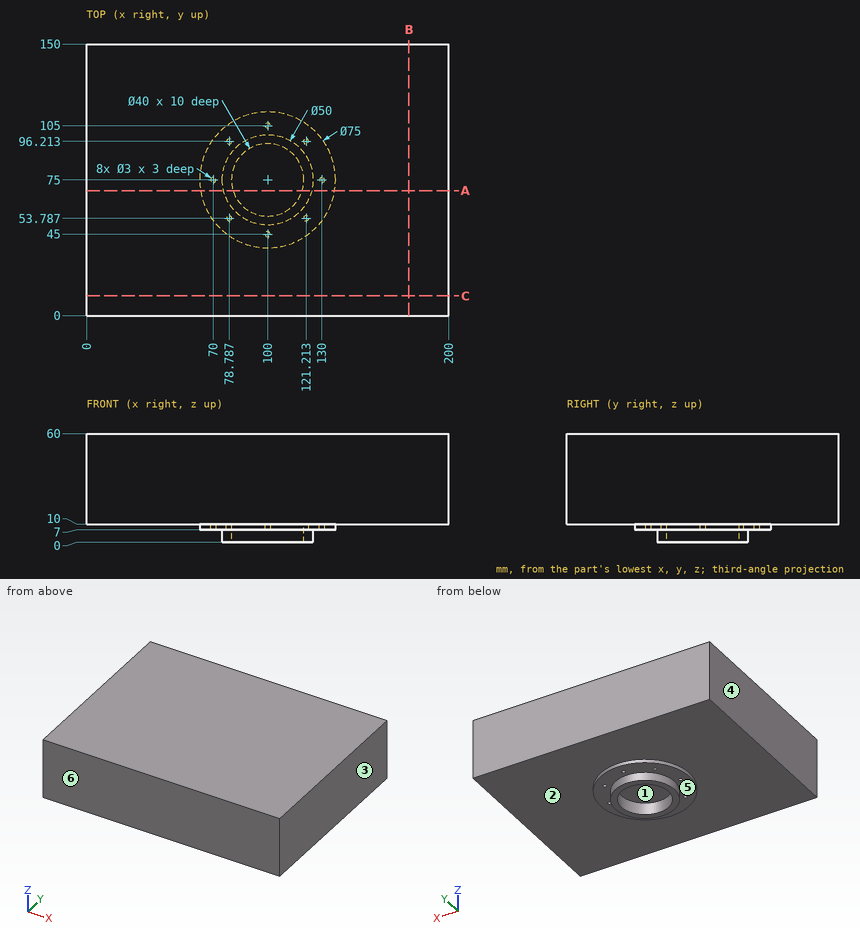
Here's the drawing with two shaded views (mm, measured from the low corner). I have some questions. A direction names the side the tool comes from. Coordinates: 2 decimals unless noted, no trailing zeros. Loops run counter-clockwise (first coordinate to the right, second up) from the corner with the lowest first, then second, coordinate; pieces in that order, holes last. Notation, with made-up numbers: (80, 59.25) -> (110, 59.25) arc R20 ccw to (110, 71.25) -> close; hole circle Ø10 at (-13, 52.5). An arc over 180 degrees is marked (long way). Use one line per item in the form item = value. Start each with the question number.
(1) If we section it at C-C (y = 11): Please give me the cut outline in (x, z).
(2) Will these pins go through, and if not, where does the flat tip stop? pin 1 (3.5 mm diameter, centred on x = 100, y = 45, fed in from -Z); pin 2 (2 mm diameter, centred on x = 105, z = 46.5, fed in from -Y); pin 3 (12 mm diameter, centred on x = 95.5, y = 78, fed in from -Z).
(3) We'd pull the mould along X, two halves only. Please class the marked faces 1, 2, 3 and 4: pulls with the +X half, pulls with the -X half, needs draft (parallel to the pull), parting line crosses it, or undercut.
(4) Please list where these lines run through material, in increasing order: line 1 along Y through (x, z) = (100, 8); line 2 along X through (y, z) = (75, 6); line 3 along Z through (x, y) = (115, 126).
(5) If we section it at B-B (x = 178): Please give me the cut outline in (y, z).
(6) If we section it at A-A (y = 69): Please give me the cut outline in (x, z), then the cut area to 3 significant figures.
(7) On a 3-axis mill with a long thin cutter (end or side, diameter ignored), from which of +Z, -Z, +X, -X, +Y, -Y can I reach the whole of each face in a straight line? I mean the marked faces 5 and 6. Say none if no direction works.
Verdict:
q1.outline = (0, 10) -> (200, 10) -> (200, 60) -> (0, 60) -> close
q2.pin_1 = 7
q2.pin_2 = 0
q2.pin_3 = 10
q3.face_1 = undercut
q3.face_2 = needs draft
q3.face_3 = pulls with the +X half
q3.face_4 = pulls with the -X half
q4.line_1 = 37.5 to 43.5, 46.5 to 55, 95 to 103.5, 106.5 to 112.5
q4.line_2 = 75 to 80, 120 to 125
q4.line_3 = 10 to 60
q5.outline = (0, 10) -> (150, 10) -> (150, 60) -> (0, 60) -> close
q6.outline = (0, 10) -> (62.98, 10) -> (62.98, 7) -> (75.73, 7) -> (75.73, 0) -> (80.92, 0) -> (80.92, 10) -> (119.08, 10) -> (119.08, 0) -> (124.27, 0) -> (124.27, 7) -> (137.02, 7) -> (137.02, 10) -> (200, 10) -> (200, 60) -> (0, 60) -> close
q6.area = 10,200 mm²
q7.face_5 = -Z
q7.face_6 = +Z, -Z, +X, -X, -Y
